Check sheet for the modelled part. Datum: model origin and axes. Units: mm. Face numbers are marked on the shaded views. A direction names the side the tool comes from. Give positions to 0.01 mm unless a question says otherwise; leave off trailing zeros. Loops run counter-clockwise (first coordinate to the right, second up) from the corner with the lowest first, then second, coordinate; pieces in that order, holes last. Notation, with made-up numbers: M 10,76.25 L 62,76.25 A17 ccw 62,80.25 Z; hole C 79,-5 d3. An arc over 180 degrees is marked long. Put each result on its own line as item: value. Start each with the question number.
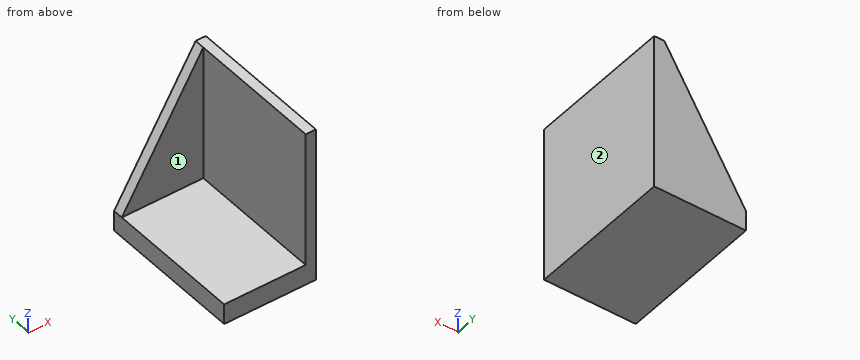
```python
from build123d import *

# Parameters (mm, degrees)
BOSS_EXTRUDE1_DEPTH = 45.475
BOSS_EXTRUDE2_DEPTH = 3.175


with BuildPart() as part:
    # Sketch1 → Boss-Extrude1 (new body)
    with BuildSketch(Plane(origin=(0, 0, 0), x_dir=(1, 0, 0), z_dir=(0, 1, 0))):
        Polygon((0, 0), (0, -48.65), (-3.175, -48.65), (-3.175, -6.35), (-28.575, -6.35), (-28.575, 0), align=None)
    extrude(amount=BOSS_EXTRUDE1_DEPTH)

    # Sketch2 → Boss-Extrude2 (add)
    with BuildSketch(Plane(origin=(0, 45.475, 0), x_dir=(1, 0, 0), z_dir=(0, 1, 0))):
        Polygon((-28.575, -6.35), (-3.175, -48.65), (-3.175, -6.35), align=None)
    extrude(amount=-BOSS_EXTRUDE2_DEPTH)


solid = part.part
```
Q1. Thickness scan on line 1 along Y through (x, z) = (-12.25, 16.5) (3 decimals); line 2 along X through (y, z) = (39, 10.5) (3 decimals); line 3 along Z through (x, y) = (-7.5, 31.5). Record the ranges inside material, lowest first. Write a range as [from, to].
Q2. Access from +Z, -Z, +X, -X, +Y, -Y to the whole of each face (thin tool, end or side, straight path). Record for the marked faces 1 and 2.
Q3. Depth check by flat-ended pin: P1, Ø5, axis at x = -14.5, y = 23.5, coming from the +Z side; P2, Ø2, axis at y = 26.5, z = 11.5, coming from the -X side (3 decimals). Enter the tip coordinate at first touch or a pass-through.
Q4. Section check A-A, the plane y = 24. Record the cut outline in (x, z) (3 decimals), then the cut area to 3 significant figures.
Q5. Section check B-B, the plane x = -19. Record the cut outline in (y, z) (3 decimals).
Found:
1. line 1: y = [42.3, 45.475]
1. line 2: x = [-3.175, 0]
1. line 3: z = [0, 6.35]
2. face 1: +Z, -X, -Y
2. face 2: +Z, -Z, +X, +Y, -Y
3. P1: stops at z = 6.35
3. P2: stops at x = -3.175
4. outline: M -28.575,0 L 0,0 L 0,48.65 L -3.175,48.65 L -3.175,6.35 L -28.575,6.35 Z
4. area: 316 mm^2
5. outline: M 0,0 L 45.475,0 L 45.475,22.296 L 42.3,22.296 L 42.3,6.35 L 0,6.35 Z
